Can you work these out from the model? Positions are in its coordinate system, mm. Face numbers are marked on the shaded views. A direction names the side the tool comes from. Round coordinates to 2 decimals unless told otherwise and drop trailing zeros. Order: outer loops, then holes, each group sorted by start corner. A loop starts at its lowest first (then second) coordinate and runs counter-clockwise, first axis right, second up.
Q1. If we section it at A-A (z = 8.25): Please give me the cut outline in (x, y), plus the area to 3 significant figures.
Q2. If we section it at C-C (y = 1.25): Please give me the cut outline in (x, z), plus the area to 3 significant figures.
Q3. If we section it at D-D (y = -2.5): Please give me the cut outline in (x, z).
Q4. Will these pins go through, and if not, where does the flat tip stop? P1, Ø5, axis at x = -0.5, y = 1, coming from the +Z side; P2, Ø1.3, axis at x = 3, z = 1.5, coming from the -Y side; P3, Ø1, axis at x = 2.5, z = 6, coming from the -Y side.
Q5. For the marked faces 1, 2, 3 and 4, which set-ups out of +Z, -Z, +X, -X, +Y, -Y let a thin tool reach every point of the face, with its end or its side?
Q6. If we section it at B-B (x = 0): Please give me the cut outline in (y, z), plus the area to 4 significant figures.
Q7. We'd pull the mould along Y, two halves only. Please class the marked faces 5, 6, 7 and 8: pulls with the +Y half, pulls with the -Y half, needs draft (parallel to the pull), parting line crosses it, or undercut.
Q8. If I drill on line 1 (X direction, y = 0.25, z = 3.75); line 2 (Y direction, x = 0, z = 4.7); line 3 (Z direction, x = -2.25, y = 1), over which ranges is the centre line in solid material (lowest first)?
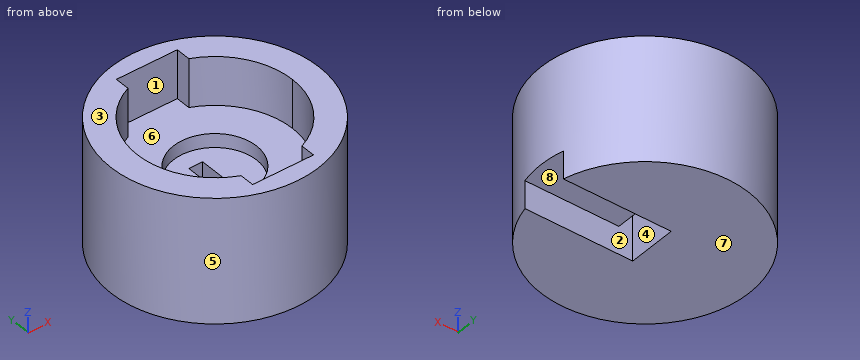
from build123d import *

# Parameters (mm, degrees)
F0_R     = 7.5
F0_W     = 1
F0_H     = 3.5
F1_DEPTH = 9
F2_W     = 3.5
F2_H     = 2
F3_DEPTH = 10
F4_W     = 1
F4_H     = 3.5
F5_DEPTH = 3.5
F6_R     = 3
F6_W     = 1
F6_H     = 3.5
F7_DEPTH = 1


with BuildPart() as f1:
    # F0 (on Top) → F1 (new body)
    with BuildSketch(Plane.XY):
        Circle(F0_R)
        Rectangle(F0_W, F0_H, mode=Mode.SUBTRACT)
    extrude(amount=F1_DEPTH)

    # F2 (on Right) → F3 (cut)
    with BuildSketch(Plane.YZ):
        with Locations((0, 1)):
            Rectangle(F2_W, F2_H)
    extrude(amount=F3_DEPTH, mode=Mode.SUBTRACT)

    # F4 (on face) → F5 (cut)
    with BuildSketch(Plane.XY.offset(9)):
        with BuildLine():
            Line((-2.2, -5.1497572758), (-2.2, 5.1497572758))
            ThreePointArc((-2.2, 5.1497572758), (-5.6, 0), (-2.2, -5.1497572758))
        make_face()
        with BuildLine():
            Line((2.2, 6.2), (-2.2, 6.2))
            Line((-2.2, 6.2), (-2.2, 5.1497572758))
            ThreePointArc((-2.2, 5.1497572758), (0, 5.6), (2.2, 5.1497572758))
            Line((2.2, 5.1497572758), (2.2, 6.2))
        make_face()
        with BuildLine():
            ThreePointArc((2.2, 5.1497572758), (0, 5.6), (-2.2, 5.1497572758))
            Line((-2.2, 5.1497572758), (-2.2, -5.1497572758))
            ThreePointArc((-2.2, -5.1497572758), (0, -5.6), (2.2, -5.1497572758))
            Line((2.2, -5.1497572758), (2.2, 5.1497572758))
        make_face()
        Rectangle(F4_W, F4_H, mode=Mode.SUBTRACT)
        with BuildLine():
            ThreePointArc((5.6, 0), (4.6733285782, 3.0854497241), (2.2, 5.1497572758))
            Line((2.2, 5.1497572758), (2.2, -5.1497572758))
            ThreePointArc((2.2, -5.1497572758), (4.6733285782, -3.0854497241), (5.6, 0))
        make_face()
        with BuildLine():
            ThreePointArc((2.2, -5.1497572758), (0, -5.6), (-2.2, -5.1497572758))
            Line((-2.2, -5.1497572758), (-2.2, -6.2))
            Line((-2.2, -6.2), (2.2, -6.2))
            Line((2.2, -6.2), (2.2, -5.1497572758))
        make_face()
    extrude(amount=-F5_DEPTH, mode=Mode.SUBTRACT)

    # F6 (on face) → F7 (cut)
    with BuildSketch(Plane.XY.offset(5.5)):
        Circle(F6_R)
        Rectangle(F6_W, F6_H, mode=Mode.SUBTRACT)
    extrude(amount=-F7_DEPTH, mode=Mode.SUBTRACT)


solid = f1.part
Solution:
1. outline: circle Ø15 at (0, 0); hole (-2.2, -6.2) - (2.2, -6.2) - (2.2, -5.15) arc R5.6 ccw to (2.2, 5.15) - (2.2, 6.2) - (-2.2, 6.2) - (-2.2, 5.15) arc R5.6 ccw to (-2.2, -5.15) - close
1. area: 71.6 mm2
2. outline: (-7.4, 0) - (-0.5, 0) - (-0.5, 4.5) - (-2.73, 4.5) - (-2.73, 5.5) - (-5.46, 5.5) - (-5.46, 9) - (-7.4, 9) - close; (0.5, 2) - (7.4, 2) - (7.4, 9) - (5.46, 9) - (5.46, 5.5) - (2.73, 5.5) - (2.73, 4.5) - (0.5, 4.5) - close
2. area: 71.2 mm2
3. outline: (-7.07, 0) - (7.07, 0) - (7.07, 9) - (5.01, 9) - (5.01, 5.5) - (1.66, 5.5) - (1.66, 4.5) - (-1.66, 4.5) - (-1.66, 5.5) - (-5.01, 5.5) - (-5.01, 9) - (-7.07, 9) - close
4. P1: stops at z = 5.5
4. P2: stops at y = -7.12
4. P3: stops at y = -7.23
5. face 1: +Z
5. face 2: -Z
5. face 3: +Z, +X, -X, +Y, -Y
5. face 4: +Z, -Z
6. outline: (-7.5, 0) - (-1.75, 0) - (-1.75, 4.5) - (-3, 4.5) - (-3, 5.5) - (-6.2, 5.5) - (-6.2, 9) - (-7.5, 9) - close; (1.75, 0) - (7.5, 0) - (7.5, 9) - (6.2, 9) - (6.2, 5.5) - (3, 5.5) - (3, 4.5) - (1.75, 4.5) - close
6. area: 69.85 mm2
7. face 5: parting line crosses it
7. face 6: undercut
7. face 7: needs draft
7. face 8: undercut
8. line 1: x = -7.5 to -0.5, 0.5 to 7.5
8. line 2: y = -7.5 to -3, 3 to 7.5
8. line 3: z = 0 to 4.5
